from build123d import *

# Parameters (mm, degrees)
SKETCH2_R           = 19.05
BOSS_EXTRUDE1_DEPTH = 62.484
SKETCH3_R           = 34.671
BOSS_EXTRUDE2_DEPTH = 12.7
SKETCH4_R           = 15.621
BOSS_EXTRUDE3_DEPTH = 19.05
SKETCH5_R           = 16.891
BOSS_EXTRUDE4_DEPTH = 2.54
FILLET1_R           = 1.524
SKETCH6_R           = 3.175
CUT_EXTRUDE1_DEPTH  = 12.7


with BuildPart() as part:
    # Sketch1 → Revolve1 (revolve)
    with BuildSketch(Plane.XY, mode=Mode.PRIVATE) as revolve1_sk:
        Polygon((0, 0), (0, 11.049), (9.722694003, 16.6624), (188.722, 16.6624), (188.722, 34.671), (201.422, 34.671), (201.422, 19.05), (300.99, 19.05), (300.99, 34.671), (326.39, 34.671), (332.329202219, 38.1), (484.729202219, 38.1), (484.729202219, 0), align=None)
    revolve(revolve1_sk.sketch.rotate(Axis((0, 0, 0), (1, 0, 0)), 90), axis=Axis((0, 0, 0), (1, 0, 0)))  # turned: the seam where the file's is

    # Sketch2 → Boss-Extrude1 (add)
    with BuildSketch(Plane(origin=(0, 0, 0), x_dir=(1, 0, 0), z_dir=(0, 1, 0))):
        with Locations(Location((251.206, 0, 0), (0, 0, 270))):  # turned: the seam where the file's is
            Circle(SKETCH2_R)
    extrude(amount=BOSS_EXTRUDE1_DEPTH)

    # Sketch3 → Boss-Extrude2 (add)
    with BuildSketch(Plane(origin=(0, 62.484, 0), x_dir=(1, 0, 0), z_dir=(0, 1, 0))):
        with Locations(Location((251.206, 0, 0), (0, 0, 270))):  # turned: the seam where the file's is
            Circle(SKETCH3_R)
    extrude(amount=-BOSS_EXTRUDE2_DEPTH)

    # Sketch4 → Boss-Extrude3 (add)
    with BuildSketch(Plane(origin=(484.729202219, 0, 0), x_dir=(0, 0, -1), z_dir=(1, 0, 0))):
        with Locations(Location((17.272, 0, 0), (0, 0, 180))):  # turned: the seam where the file's is
            Circle(SKETCH4_R)
    extrude(amount=BOSS_EXTRUDE3_DEPTH)

    # Sketch5 → Boss-Extrude4 (add)
    with BuildSketch(Plane(origin=(484.729202219, 0, 0), x_dir=(0, 0, -1), z_dir=(1, 0, 0))):
        with Locations(Location((-19.812, 0, 0), (0, 0, 180))):  # turned: the seam where the file's is
            Circle(SKETCH5_R)
    extrude(amount=BOSS_EXTRUDE4_DEPTH)

    # Fillet1
    fillet1_edges = [part.edges().sort_by_distance(p)[0] for p in [
        (9.722694003, 0, -16.6624),
        (0, 0, -11.049),
    ]]
    fillet(fillet1_edges, radius=FILLET1_R)

    # Sketch6 → Cut-Extrude1 (cut)
    with BuildSketch(Plane.ZY):
        Circle(SKETCH6_R)
    extrude(amount=-CUT_EXTRUDE1_DEPTH, mode=Mode.SUBTRACT)


solid = part.part
Could you check a few things on this model? Use its own coordinates, in mm. A direction names the side the tool comes from. Give positions to 0.01 mm unless a question says otherwise; leave off trailing zeros. Order: outer loops, then holes, each group sorted by start corner. A loop starts at its lowest first (then second) coordinate and runs counter-clockwise, first axis right, second up.
1. For faces 5 (the cylindrical face through (217.36, 56.22, -7.52)), 6 (the cylindrical face through (100.677, -5.005, 15.893)), 7 (the flat face through (236, 49.784, 15)), 8 (the flat face through (503.779, 0, -17)), 9 (the cylindrical face through (485.981, 6.469, 35.415)), which set-ups out of +Z, -Z, +X, -X, +Y, -Y let a thin tool reach every point of the face, with its end or its side?
2. I need wall thicknesses on L1, parallel to X at y = -12, z = -19; L2, parallel to X at y = -29, z = 9.5; L3, parallel to Z at x = 228.5, y = -9. Which ranges of each line are inside material? Lowest first, please.
3. Will these pins go through, and if not, where does the flat tip stop? P1, Ø2, axis at y = -8.5, z = -30.5, coming from the +X side; P2, Ø10, axis at x = 147.5, z = 6.5, coming from the -Y side; P3, Ø12, axis at x = 351.5, y = -7, coming from the +Z side; P4, Ø8, axis at x = 257.5, y = 6, coming from the +Z side.
4. We'd pull the mould along X, two halves only. Please class faces 1 (the flat face through (188.722, -8, -15)), 2 (the flat face through (252, 62.484, 0)), 3 (the cylindrical face through (252.04, 30.08, -19.03)), 4 (the conical face through (326.762, -29.416, 18.754)): pulls with the +X half, pulls with the -X half, needs draft (parallel to the pull), parting line crosses it, or undercut.
5. Suppose I cut it at A-A (x = 320). List the corners of the cut face in (y, z) for me, plus the area to 3 significant figures.
6. Suppose I cut it at B-B (x = 84.5). List the corners of the cut face in (y, z) for me, plus the area to 3 significant figures.
Solved:
1. face 5: +Y
1. face 6: -X
1. face 7: none
1. face 8: +Z, -Z, +X, +Y, -Y
1. face 9: +X
2. L1: x = 188.72 to 201.42, 300.99 to 503.78
2. L2: x = 188.72 to 201.42, 300.99 to 484.73
2. L3: z = -16.79 to 16.79
3. P1: stops at x = 503.78
3. P2: stops at y = -16.59
3. P3: stops at z = 38.09
3. P4: stops at z = 18.94
4. face 1: pulls with the -X half
4. face 2: needs draft
4. face 3: undercut
4. face 4: undercut
5. outline: circle Ø69.34 at (0, 0)
5. area: 3,780 mm2
6. outline: circle Ø33.32 at (0, 0)
6. area: 872 mm2
